The model under review builds one solid part; all positions refer to its coordinate system, in mm. A direction names the side the tool comes from. Coordinates: 2 decimals unless noted, no trailing zeros. Write each loop counter-clockwise with the first axis right and the second up, starting at its lowest first coordinate (ties: lowest second). Pieces come first, ordered by that corner, then holes.
```python
from build123d import *
from build123d.topology import SkipClean

# Parameters (mm, degrees)
SKETCH_1_W               = 159
SKETCH_1_H               = 159
EXTRUDE_1_DEPTH          = 5
SKETCH_2_R               = 2
CUT_EXTRUDE_1_DEPTH      = 5.1
SKETCH_3_R               = 3.65
CUT_EXTRUDE_2_DEPTH      = 4.05
EXTRUDE_3_DEPTH          = 60
SKETCH_6_R               = 3.175
CUT_EXTRUDE_3_DEPTH      = 60
SKETCH_7_R               = 4.9
CUT_EXTRUDE_4_DEPTH      = 4
SKETCH_8_W               = 110.4
SKETCH_8_H               = 88.4
CUT_EXTRUDE_5_DEPTH      = 3
SKETCH_9_R               = 1.5
CUT_EXTRUDE_6_DEPTH      = 10
FILLET_1_R               = 10
FILLET_2_R               = 10
FILLET_3_R               = 10
FILLET_4_R               = 10
SKETCH_11_W              = 49.5
SKETCH_11_H              = 5
EXTRUDE_4_DEPTH          = 60
SKETCH_12_W              = 49.5
SKETCH_12_H              = 5
EXTRUDE_5_DEPTH          = 60
SKETCH_13_R              = 1.5
CUT_EXTRUDE_7_DEPTH      = 5
SKETCH_14_R              = 3
CUT_EXTRUDE_8_DEPTH      = 2.5
SKETCH_16_R              = 1.5
EXTRUDE_6_DEPTH          = 0.5
SKETCH_16_R_2            = 1.448084079
EXTRUDE_6_2_DEPTH        = 0.5
EXTRUDE_6_3_DEPTH        = 0.5
EXTRUDE_6_4_DEPTH        = 0.5
SKETCH_18_W              = 110.4
SKETCH_18_H              = 88.4
EXTRUDE_7_DEPTH          = 3
SKETCH_18_2_W            = 110.4
SKETCH_18_2_H            = 88.4
EXTRUDE_8_DEPTH          = 2
SKETCH_22_W              = 104
SKETCH_22_H              = 91
CUT_EXTRUDE_10_DEPTH     = 3
SKETCH_23_R              = 1.5
CUT_EXTRUDE_11_DEPTH     = 2
CUT_EXTRUDE_12_OUTLINE_R = 1.5
CUT_EXTRUDE_12_DEPTH     = 3


# Read off the part's stored shape, not the designer's step: the extrude step
with BuildPart() as part:
    # Sketch 1 → Extrude 1 (new body)
    with BuildSketch(Plane(origin=(0, 0, 0), x_dir=(1, 0, 0), z_dir=(0, 1, 0))):
        with Locations((-0.471002014, -22.874671738)):
            Rectangle(SKETCH_1_W, SKETCH_1_H)
    extrude(amount=EXTRUDE_1_DEPTH)

    # Sketch 2 → Cut-Extrude 1 (cut)
    with BuildSketch(Plane(origin=(0, 5, 0), x_dir=(1, 0, 0), z_dir=(0, 1, 0))):
        with Locations(Location((-69.971002014, -77.374671738, 0), (0, 0, 270))):
            Circle(SKETCH_2_R)
        with Locations(Location((-69.971002014, 31.625328262, 0), (0, 0, 270))):
            Circle(SKETCH_2_R)
        with Locations(Location((69.028997986, -77.374671738, 0), (0, 0, 270))):
            Circle(SKETCH_2_R)
        with Locations(Location((69.028997986, 31.625328262, 0), (0, 0, 270))):
            Circle(SKETCH_2_R)
    extrude(amount=-CUT_EXTRUDE_1_DEPTH, mode=Mode.SUBTRACT)

    # Sketch 3 → Cut-Extrude 2 (cut)
    with BuildSketch(Plane(origin=(0, 5, 0), x_dir=(1, 0, 0), z_dir=(0, 1, 0))):
        with Locations(Location((-69.971002014, -77.374671738, 0), (0, 0, 270))):
            Circle(SKETCH_3_R)
        with Locations(Location((69.028997986, -77.374671738, 0), (0, 0, 270))):
            Circle(SKETCH_3_R)
        with Locations(Location((69.028997986, 31.625328262, 0), (0, 0, 270))):
            Circle(SKETCH_3_R)
        with Locations(Location((-69.971002014, 31.625328262, 0), (0, 0, 270))):
            Circle(SKETCH_3_R)
    extrude(amount=-CUT_EXTRUDE_2_DEPTH, mode=Mode.SUBTRACT)

    # Sketch 4 → Extrude 3 (add)
    with BuildSketch(Plane.XY.offset(102.374671738)):
        Polygon((19.528997986, 5), (-0.471002014, 5), (-20.471002014, 5), (-20.471002014, 0), (19.528997986, 0), align=None)
    extrude(amount=EXTRUDE_3_DEPTH)

    # Sketch 6 → Cut-Extrude 3 (cut)
    with BuildSketch(Plane.XZ):
        with Locations(Location((-0.471002014, 145.374671738, 0), (0, 0, 270))):
            Circle(SKETCH_6_R)
    extrude(amount=-CUT_EXTRUDE_3_DEPTH, mode=Mode.SUBTRACT)

    # Sketch 7 → Cut-Extrude 4 (cut)
    with BuildSketch(Plane(origin=(0, 0, 0), x_dir=(-1, 0, 0), z_dir=(0, -1, 0))):
        with Locations(Location((0.471002014, -145.374671738, 0), (0, 0, 90))):
            Circle(SKETCH_7_R)
    extrude(amount=-CUT_EXTRUDE_4_DEPTH, mode=Mode.SUBTRACT)

    # Sketch 8 → Cut-Extrude 5 (cut)
    with BuildSketch(Plane(origin=(0, 5, 0), x_dir=(1, 0, 0), z_dir=(0, 1, 0))):
        with Locations((-0.471002014, 10.625328262)):
            Rectangle(SKETCH_8_W, SKETCH_8_H)
    extrude(amount=-CUT_EXTRUDE_5_DEPTH, mode=Mode.SUBTRACT)

    # Sketch 9 → Cut-Extrude 6 (cut)
    with BuildSketch(Plane(origin=(0, 2, 0), x_dir=(1, 0, 0), z_dir=(0, 1, 0))):
        with Locations(Location((52.028997986, 52.125328262, 0), (0, 0, 270))):
            Circle(SKETCH_9_R)
        with Locations(Location((52.028997986, -30.874671738, 0), (0, 0, 270))):
            Circle(SKETCH_9_R)
        with Locations(Location((-52.971002014, -30.874671738, 0), (0, 0, 270))):
            Circle(SKETCH_9_R)
        with Locations(Location((-52.971002014, 52.125328262, 0), (0, 0, 270))):
            Circle(SKETCH_9_R)
    extrude(amount=-CUT_EXTRUDE_6_DEPTH, mode=Mode.SUBTRACT)

    # Fillet 1
    fillet_1_edges = [part.edges().sort_by_distance(p)[0] for p in [
        (79.028997986, 2.5, -56.625328262),
    ]]
    fillet(fillet_1_edges, radius=FILLET_1_R)

    # Fillet 2
    fillet_2_edges = [part.edges().sort_by_distance(p)[0] for p in [
        (-79.971002014, 2.5, -56.625328262),
    ]]
    fillet(fillet_2_edges, radius=FILLET_2_R)

    # Fillet 3
    fillet_3_edges = [part.edges().sort_by_distance(p)[0] for p in [
        (-79.971002014, 2.5, 102.374671738),
    ]]
    fillet(fillet_3_edges, radius=FILLET_3_R)

    # Fillet 4
    fillet_4_edges = [part.edges().sort_by_distance(p)[0] for p in [
        (79.028997986, 2.5, 102.374671738),
    ]]
    fillet(fillet_4_edges, radius=FILLET_4_R)

    # Sketch 11 → Extrude 4 (add)
    with BuildSketch(Plane.XY.offset(102.374671738)):
        with Locations((-45.221002014, 2.5)):
            Rectangle(SKETCH_11_W, SKETCH_11_H)
    extrude(amount=EXTRUDE_4_DEPTH)

    # Sketch 12 → Extrude 5 (add)
    with BuildSketch(Plane.XY.offset(102.374671738)):
        with Locations((44.278997986, 2.5)):
            Rectangle(SKETCH_12_W, SKETCH_12_H)
    extrude(amount=EXTRUDE_5_DEPTH)

    # Sketch 13 → Cut-Extrude 7 (cut)
    with BuildSketch(Plane(origin=(0, 5, 0), x_dir=(1, 0, 0), z_dir=(0, 1, 0))):
        with Locations(Location((-25, -80, 0), (0, 0, 270))):
            Circle(SKETCH_13_R)
        with Locations(Location((-25, -154, 0), (0, 0, 270))):
            Circle(SKETCH_13_R)
        with Locations(Location((25, -80, 0), (0, 0, 270))):
            Circle(SKETCH_13_R)
        with Locations(Location((25, -154, 0), (0, 0, 270))):
            Circle(SKETCH_13_R)
    extrude(amount=-CUT_EXTRUDE_7_DEPTH, mode=Mode.SUBTRACT)

    # Sketch 14 → Cut-Extrude 8 (cut)
    with BuildSketch(Plane.XZ):
        with Locations(Location((-25, 80, 0), (0, 0, 270))):
            Circle(SKETCH_14_R)
        with Locations(Location((-25, 154, 0), (0, 0, 270))):
            Circle(SKETCH_14_R)
        with Locations(Location((25, 154, 0), (0, 0, 270))):
            Circle(SKETCH_14_R)
        with Locations(Location((25, 80, 0), (0, 0, 270))):
            Circle(SKETCH_14_R)
    extrude(amount=-CUT_EXTRUDE_8_DEPTH, mode=Mode.SUBTRACT)



with BuildPart() as body_2:
    # Sketch 16 → Extrude 6 (new body)
    with BuildSketch(Plane(origin=(0, 2, 0), x_dir=(1, 0, 0), z_dir=(0, 1, 0))):
        with Locations(Location((-52.971002014, 52.125328262, 0), (0, 0, 270))):
            Circle(SKETCH_16_R)
    extrude(amount=EXTRUDE_6_DEPTH)


with BuildPart() as body_3:
    # Sketch 16 → Extrude 6 2 (new body)
    with BuildSketch(Plane(origin=(0, 2, 0), x_dir=(1, 0, 0), z_dir=(0, 1, 0))):
        with Locations(Location((52.028997986, 52.125328262, 0), (0, 0, 270))):
            Circle(SKETCH_16_R_2)
    extrude(amount=EXTRUDE_6_2_DEPTH)


with BuildPart() as body_4:
    # Sketch 16 → Extrude 6 3 (new body)
    with BuildSketch(Plane(origin=(0, 2, 0), x_dir=(1, 0, 0), z_dir=(0, 1, 0))):
        with Locations(Location((-52.971002014, -30.874671738, 0), (0, 0, 270))):
            Circle(SKETCH_16_R)
    extrude(amount=EXTRUDE_6_3_DEPTH)


with BuildPart() as body_5:
    # Sketch 16 → Extrude 6 4 (new body)
    with BuildSketch(Plane(origin=(0, 2, 0), x_dir=(1, 0, 0), z_dir=(0, 1, 0))):
        with Locations(Location((52.028997986, -30.874671738, 0), (0, 0, 270))):
            Circle(SKETCH_16_R)
    extrude(amount=EXTRUDE_6_4_DEPTH)


with BuildPart() as part_1:
    add(part.part)

    add(body_2.part)  # Extrude 7 merges body 2

    add(body_3.part)  # Extrude 7 merges body 3

    add(body_4.part)  # Extrude 7 merges body 4

    add(body_5.part)  # Extrude 7 merges body 5
    # Sketch 18 → Extrude 7 (add)
    with BuildSketch(Plane(origin=(0, 2, 0), x_dir=(1, 0, 0), z_dir=(0, 1, 0))):
        with Locations((-0.471002014, 10.625328262)):
            Rectangle(SKETCH_18_W, SKETCH_18_H)
    extrude(amount=EXTRUDE_7_DEPTH)

    # Sketch 18_2 → Extrude 8 (add)
    with BuildSketch(Plane(origin=(0, 2, 0), x_dir=(1, 0, 0), z_dir=(0, 1, 0))):
        with Locations((-0.471002014, 10.625328262)):
            Rectangle(SKETCH_18_2_W, SKETCH_18_2_H)
    extrude(amount=-EXTRUDE_8_DEPTH)

    # Sketch 22 → Cut-Extrude 10 (cut)
    with BuildSketch(Plane(origin=(0, 5, 0), x_dir=(1, 0, 0), z_dir=(0, 1, 0))):
        with Locations((0, 9.5)):
            Rectangle(SKETCH_22_W, SKETCH_22_H)
    extrude(amount=-CUT_EXTRUDE_10_DEPTH, mode=Mode.SUBTRACT)

    # Sketch 23 → Cut-Extrude 11 (cut)
    with BuildSketch(Plane(origin=(0, 5, 0), x_dir=(1, 0, 0), z_dir=(0, 1, 0))):
        with Locations(Location((-54.5, 40, 0), (0, 0, 270))):
            Circle(SKETCH_23_R)
        with Locations(Location((54.5, 40, 0), (0, 0, 270))):
            Circle(SKETCH_23_R)
        with Locations(Location((-54.5, -20, 0), (0, 0, 270))):
            Circle(SKETCH_23_R)
        with Locations(Location((54.5, -20, 0), (0, 0, 270))):
            Circle(SKETCH_23_R)
    extrude(amount=-CUT_EXTRUDE_11_DEPTH, mode=Mode.SUBTRACT)

    # Cut-Extrude 12 outline → Cut-Extrude 12 (cut)
    with SkipClean():  # the faces are left unmerged after this step: merging them gives an invalid solid
        with BuildSketch(Plane(origin=(0, 0, 0), x_dir=(1, 0, 0), z_dir=(0, 1, 0))):
            with Locations((-54.5, 40)):
                Circle(CUT_EXTRUDE_12_OUTLINE_R)
            with Locations((54.5, -20)):
                Circle(CUT_EXTRUDE_12_OUTLINE_R)
            with Locations((-54.5, -20)):
                Circle(CUT_EXTRUDE_12_OUTLINE_R)
            with Locations((54.5, 40)):
                Circle(CUT_EXTRUDE_12_OUTLINE_R)
        extrude(amount=CUT_EXTRUDE_12_DEPTH, mode=Mode.SUBTRACT)


solid = part_1.part
```
Item 1: Take a section at A-A, the plane z = -7.5. Write out the cut boundary in (x, y), plus the area to 3 significant figures.
Solved:
outline: (-79.97, 0) - (79.03, 0) - (79.03, 5) - (52, 5) - (52, 2) - (-52, 2) - (-52, 5) - (-79.97, 5) - close
area: 483 mm2
Item 2: For pin 1 (5 mm diameter, centred on x = -54.5, z = 20, fed in from +Y); pin 2 (1.8 mm diameter, centred on x = 25.5, z = 154.5, fed in from -Y); pin 3 (7.5 mm diameter, centred on x = -0.47, z = 145.37, fed in from -Y); pin 4 (2.5 mm diameter, centred on y = 2.5, z = 121, fed in from +X), all flat-tipped, find the tip position at first contact; note any pin that passes through.
Solved:
pin 1: stops at y = 5
pin 2: stops at y = 2.5
pin 3: stops at y = 4
pin 4: stops at x = 69.03
Item 3: Mouldability with a two-part tool opening along Z and no side actions: class faces 1 (the face through (76.022, 2.535, -53.774)), 2 (the face through (-0.331, 4.493, 148.547)), 3 (the face through (69.029, 2, 132)) as pulls with the +Z half, pulls with the -Z half, needs draft (parallel to the pull), parting line crosses it, or undercut.
Solved:
face 1: pulls with the -Z half
face 2: undercut
face 3: needs draft
Item 4: Take a section at B-B, the plane x = 49.5. Write out the cut boundary in (y, z), plus the area to 3 significant figures.
Solved:
outline: (0, -56.63) - (5, -56.63) - (5, -55) - (2, -55) - (2, 36) - (5, 36) - (5, 162.37) - (0, 162.37) - close
area: 822 mm2
Item 5: To check wall thickness, follow line 1 along Z through (x, y) = (54.5, 0.65); line 2 along X through (y, z) = (4.05, -40); line 3 along Z through (x, y) = (-70.5, 2.35). State the ranges of each line that lie inside material, in increasing order.
Solved:
line 1: z = -56.63 to -41.5, -38.5 to 18.5, 21.5 to 162.37
line 2: x = -79.97 to -56, -53 to -52, 52 to 53, 56 to 79.03
line 3: z = -56.61 to -35.24, -28.01 to 73.76, 80.99 to 102.36
Item 6: Take a section at C-C, the plane z = 107.5. Write out the cut boundary in (x, y).
Solved:
outline: (-69.97, 0) - (69.03, 0) - (69.03, 5) - (-69.97, 5) - close
Item 7: Machinability: for faces 4 (the face through (-1, 3, 162.375)), 5 (the face through (-73.21, 3, 79.06)), 6 (the face through (1, 2, 140.7)), which of the approach directions +Z, -Z, +X, -X, +Y, -Y give a long, thin tool a straight path to every point of the face, cutting with its end or side? Answer none if there is none.
Solved:
face 4: +Z, +X, -X, +Y, -Y
face 5: +Y
face 6: -Y
